Autodesk Inventor part; units mm, degrees
ref_plane "YZ Plane" through (0, 0, 0) normal (1, 0, 0) x (0, 1, 0)
ref_plane "XZ Plane" through (0, 0, 0) normal (0, 1, 0) x (-1, 0, 0)
ref_plane "XY Plane" through (0, 0, 0) normal (0, 0, 1) x (1, 0, 0)
sketch "Sketch1" plane through (0, 0, 0) normal (0, 0, 1) x (1, 0, 0)
  point P0 (0, 0)
sketch "Sketch2" plane through (0, 0, 0) normal (0, 0, 1) x (1, 0, 0)
  line L0 (0, 0) -> (335, 0)
  line L1 (335, 0) -> (335, 450)
  line L2 (335, 450) -> (0, 450)
  line L3 (0, 450) -> (0, 0)
  line L4 (0, 0) -> (167.5, 0)
  dimension "d0" = 335
  dimension "d1" = 450
  dimension "d2" = 167.5
extrude "Extrusion1" add sketch "Sketch2" along normal blind 7
sketch "Sketch3" plane through (0, 0, 7) normal (0, 0, 1) x (1, 0, 0)
  line L0 (0, 0) -> (167.5, 0)
  line L1 (0, 0) -> (335, 0)
  line L2 (167.5, 0) -> (167.5, 450)
  line L3 (335, 450) -> (0, 450)
  line L4 (0, 0) -> (0, 325)
  line L5 (0, 450) -> (0, 0)
  line L6 (0, 325) -> (335, 325)
  line L7 (335, 0) -> (335, 450)
  line L8 (335, 325) -> (167.5, 450)
  line L9 (167.5, 450) -> (0, 325)
  dimension "d5" = 167.5
  dimension "d6" = 325
extrude "Extrusion2" cut sketch "Sketch3" against normal blind 166.0375 contours L5 L3 L9
sketch "Sketch5" plane through (0, 0, 7) normal (0, 0, 1) x (1, 0, 0)
  line L0 (167.5, 450) -> (335, 450)
  line L1 (335, 450) -> (167.5, 450)
  line L2 (335, 450) -> (335, 0)
  line L3 (335, 0) -> (335, 450)
  line L4 (335, 0) -> (335, 325)
  line L5 (167.5, 450) -> (335, 325)
  line L6 (335, 450) -> (167.5, 450)
  line L7 (335, 325) -> (335, 450)
  point P0 (0, 0)
  dimension "d10" = 325
extrude "Extrusion3" cut sketch "Sketch5" against normal blind 305.45
sketch "Sketch11" plane through (0, 0, 7) normal (0, 0, 1) x (1, 0, 0)
  line L0 (0, 325) -> (335, 325)
  line L1 (335, 325) -> (167.5, 325)
  line L2 (167.5, 325) -> (167.5, 276)
  line L3 (167.5, 276) -> (167.5, 195)
  line L4 (167.5, 195) -> (167.5, 235.5)
  circle A0 centre (167.5, 235.5) radius 40.5
  point P0 (0, 0)
  dimension "d29" = 49
  dimension "d30" = 81
extrude "Extrusion6" cut sketch "Sketch11" against normal blind 10
properties part number "fundo" material "Polycarbonate, Clear"
Model file for the job. Use its own axes, mm. Round coordinates to 2 decimals unless told otherwise and drop trailing zeros. Write each loop counter-clockwise with the first axis right and the second up, starting at its lowest first coordinate (ties: lowest second). Pieces come first, ordered by that corner, then holes. Notation, with made-up numbers: (-17, -2.5) - (12, -2.5) arc R13 ccw to (12, 5.5) - close; hole circle Ø4 at (58, 50.5). An arc over 180 degrees is marked (long way). One line per item, written item: value.
(1) Cut at A-A, the plane y = 235.5. Give the cut face in (x, z).
Values follow:
outline: (0, 0) - (127, 0) - (127, 7) - (0, 7) - close; (208, 0) - (335, 0) - (335, 7) - (208, 7) - close
(2) Two-plate mould, pull along X, no slides. Class faces 1 (the flat face through (165, 178, 0)), 2 (the cylindrical face through (158.72, 195.963, 3.549)), 3 (the flat face through (84.923, 388.375, 3.549)): pulls with the +X half, pulls with the -X half, needs draft (parallel to the pull), parting line crosses it, or undercut.
Values follow:
face 1: needs draft
face 2: undercut
face 3: pulls with the -X half
(3) Cut at B-B, the plane z = 2. Give the cut face in (x, y).
Values follow:
outline: (0, 0) - (335, 0) - (335, 325) - (167.5, 450) - (0, 325) - close; hole circle Ø81 at (167.5, 235.5)
(4) Cut at D-D, the plane y = 415. Give the cut face in (x, z).
Values follow:
outline: (120.6, 0) - (214.4, 0) - (214.4, 7) - (120.6, 7) - close
(5) Cut at C-C, the plane x = 160.5. Give the cut face in (y, z), plus the area to 3 significant figures.
Values follow:
outline: (0, 0) - (195.61, 0) - (195.61, 7) - (0, 7) - close; (275.39, 0) - (444.78, 0) - (444.78, 7) - (275.39, 7) - close
area: 2,550 mm²
(6) Wall check: probe 1 along X at (y, z) = (235.5, 4); probe 2 along Y at (x, z) = (167.5, 3.25); probe 3 along X at (y, z) = (217, 0.75). Give the ranges that are in metal, low to high.
Values follow:
probe 1: x = 0 to 127, 208 to 335
probe 2: y = 0 to 195, 276 to 450
probe 3: x = 0 to 131.47, 203.53 to 335
(7) Drop flat-ended pins along their axis: P1, Ø3, axis at y = 403, z = 4, coming from the +X side; P2, Ø1.5, axis at x = 206, y = 103, coming from the -Z side; P3, Ø1, axis at y = 403.5, z = 1.5, coming from the +X side. Give the stop position or say it passes through.
Values follow:
P1: stops at x = 232.49
P2: stops at z = 0
P3: stops at x = 230.48
